Input: part model. Units: mm. Frame: model coordinates. A direction names the side the tool comes from. Coordinates: 2 decimals unless noted, no trailing zeros. Write each loop counter-clockwise with the first axis right and the second up, starting at its lowest first coordinate (ties: lowest second). Pieces come first, ordered by that corner, then holes. Notation, with made-up numbers: M 20.5,13 L 63.5,13 A6 ccw 63.5,22 Z; hole C 89.5,73 d2. An arc over 180 degrees is marked long. Use CSV: the item, a comma, the result in double quotes.
Solid Edge part; units mm, degrees
sketch "Sketch1" plane through (0, 0, 0) normal (0, -1, 0) x (1, 0, 0)
  line L0 (-67.5, -31.25) -> (67.5, -31.25)
  line L1 (67.5, -31.25) -> (67.5, 31.25)
  line L2 (67.5, 31.25) -> (-67.5, 31.25)
  line L3 (-67.5, 31.25) -> (-67.5, -31.25)
  dimension "D1" = 67.5
  dimension "D2" = 67.5
extrude "Protrusion1" add sketch "Sketch1" against normal blind 18
hole "Hole_1" at (-0.3, 18, -11.35) direction (0, -1, 0) diameter 18.5 end through all
hole "Hole1" at (-23.7, 18, -11.35) direction (0, -1, 0) diameter 18.5 end through all
hole "Hole_3" at (13.05, 18, 1.25) direction (0, -1, 0) diameter 2.5 depth 8
hole "Hole2" at (13.05, 18, -23.75) direction (0, -1, 0) diameter 2.5 depth 8
hole "Hole3" at (-36.95, 18, -23.75) direction (0, -1, 0) diameter 2.5 depth 8
hole "Hole4" at (-36.95, 18, 1.25) direction (0, -1, 0) diameter 2.5 depth 8
hole "Hole_7" at (-0.3, 9, 31.25) direction (0, 0, -1) diameter 4 end up to next
hole "Hole5" at (-23.7, 9, 31.25) direction (0, 0, -1) diameter 4 end up to next
sketch "Sketch2" plane through (0, 9, 31.25) normal (0, 0, 1) x (-1, 0, 0)
  line L0 (-8.95, -3) -> (67.5, -3)
  arc A0 (67.5, 3) -> (67.5, -3) centre (67.5, 0) cw
  line L1 (-8.95, 3) -> (67.5, 3)
  arc A1 (-8.95, -3) -> (-8.95, 3) centre (-8.95, 0) cw
extrude "ExtrudedCutout_2" cut sketch "Sketch2" against normal blind 20
hole "Hole_9" at (-23.7, 9, 11.25) direction (0, 0, -1) diameter 6 depth 2
hole "Hole6" at (-0.3, 9, 11.25) direction (0, 0, -1) diameter 6 depth 2
fillet "Round_1" radius 1.5 4 edges at (67.5, 18, 0) (67.5, 0, 0) (-67.5, 18, 0) (-67.5, 0, 0)
hole "Hole_11" at (50, 9, -31.25) direction (0, 0, 1) diameter 3.3 depth 15 tip angle 118
hole "Hole7" at (-50, 9, -31.25) direction (0, 0, 1) diameter 3.3 depth 15 tip angle 118
hole "Hole8" at (22.5, 9, -31.25) direction (0, 0, 1) diameter 3.3 depth 15 tip angle 118
hole "Hole9" at (-12.5, 9, -31.25) direction (0, 0, 1) diameter 3.3 depth 15 tip angle 118
hole "Hole_15" at (12.5, 14.5, 31.25) direction (0, 0, -1) diameter 2.5 depth 8
hole "Hole10" at (12.5, 3.5, 31.25) direction (0, 0, -1) diameter 2.5 depth 8
hole "Hole11" at (-62.5, 3.5, 31.25) direction (0, 0, -1) diameter 2.5 depth 8
hole "Hole12" at (-62.5, 14.5, 31.25) direction (0, 0, -1) diameter 2.5 depth 8
hole "Hole_19" at (8.9, 0, 17.25) direction (0, 1, 0) diameter 2.5 depth 8
hole "Hole13" at (-21.1, 0, 17.25) direction (0, 1, 0) diameter 2.5 depth 8
hole "Hole_21" at (-1.45, 18, 18.25) direction (0, -1, 0) diameter 5 end up to next
hole "Hole14" at (-7.95, 18, 18.25) direction (0, -1, 0) diameter 5 end up to next
hole "Hole15" at (-24.85, 18, 18.25) direction (0, -1, 0) diameter 5 end up to next
hole "Hole16" at (-31.35, 18, 18.25) direction (0, -1, 0) diameter 5 end up to next
properties material "Acrylic, high impact grade"
1. Mould query, pull axis X, two halves, no side actions, for faces 1 (the flat face through (-12, 9, 11.25)), 2 (the flat face through (-63, 15, 23.25)). Classes: pulls with the +X half, pulls with the -X half, needs draft (parallel to the pull), parting line crosses it, or undercut.
Resolved:
face 1,"needs draft"
face 2,"undercut"
2. Material intervals for line 1 (X direction, y = 14.65, z = 18.25); line 2 (X direction, y = 12.25, z = -11); line 3 (X direction, y = 9.25, z = 7), sorted ascending. Write a range as [from, to].
Resolved:
line 1,"x = [-67.5, -33.85], [-28.85, -27.35], [-22.35, -10.45], [-5.45, -3.95], [1.05, 67.5]"
line 2,"x = [-67.5, -32.94], [-14.46, -9.54], [8.94, 67.5]"
line 3,"x = [-67.5, -25.68], [-21.72, -2.28], [1.68, 67.5]"
3. Section C-C (y = 14.5). State how many separate pieces and enclosed holes the cut face has, then the cut area to 3 significant figures.
Resolved:
separate pieces,"1"
enclosed holes,"10"
area,"7,760 mm^2"
4. Access query for faces 3 (the cylindrical face through (48.61, 9.89, -23.64)), 4 (the flat face through (2, 8, 9.25)), 5 (the cylindrical face through (11.996, 13.944, -23.078)). Directions: +Z, -Z, +X, -X, +Y, -Y. A direction counts if a zero-diameter tool reaches every point of the face in a straight line with its end or side. Return the directions, or none.
Resolved:
face 3,"-Z"
face 4,"+Z"
face 5,"+Y"
5. Section B-B (x = -40.5). Return loops of the section in (y, z).
Resolved:
outline,"M 0,-31.25 L 18,-31.25 L 18,31.25 L 12,31.25 L 12,11.25 L 6,11.25 L 6,31.25 L 0,31.25 Z"
6. Contact query for flat-ended pins moving along their axis: pin 1 Ø2 at (x, y) = (-50, 9) entering from -Z; pin 2 Ø3.5 at (x, y) = (-23.7, 9) entering from +Z; pin 3 Ø3 at (x, y) = (-12.5, 9) entering from -Z. Output: stop coordinate, or through.
Resolved:
pin 1,"stops at z = -15.86"
pin 2,"stops at z = -20.43"
pin 3,"stops at z = -16.16"
7. Section A-A (z = -11.35). Return loops of the section in (x, y), then the cut area to 3 significant figures.
Resolved:
outline,"M -67.5,1.5 A1.5 ccw -66,0 L -32.95,0 L -32.95,18 L -66,18 A1.5 ccw -67.5,16.5 Z; M -14.45,0 L -9.55,0 L -9.55,18 L -14.45,18 Z; M 8.95,0 L 66,0 A1.5 ccw 67.5,1.5 L 67.5,16.5 A1.5 ccw 66,18 L 8.95,18 Z"
area,"1,760 mm^2"
